Model file for the job. Use its own axes, mm. Face numbers are marked on the shaded views. A direction names the side the tool comes from. Coordinates: 2 decimals unless noted, no trailing zeros. Order: outer loops, then holes, each group sorted by start corner. A loop starts at its lowest first (then second) coordinate and runs counter-clockwise, first axis right, second up. Notation, with made-up numbers: (3.25, 39.5) - (38.25, 39.5) arc R21 cw to (38.25, 43.5) - close; hole circle Ø4 at (24, -4.5). An arc over 180 degrees is marked (long way). Put each result on its own line as item: value. Start each with the question number.
```python
from build123d import *

# Parameters (mm, degrees)
SKETCH1_R           = 11.1125
SKETCH1_R_2         = 4.7625
SKETCH1_R_3         = 14.2875
BOSS_EXTRUDE1_DEPTH = 76.2


with BuildPart() as part:
    # Sketch1 → Boss-Extrude1 (new body)
    with BuildSketch(Plane.XY):
        Polygon((-101.6, 0), (101.6, 0), (130.929393675, 50.8), (130.929393675, 127), (118.229393675, 127), (25.4, 50.8), (-25.4, 50.8), (-118.229393675, 127), (-130.929393675, 127), (-130.929393675, 50.8), align=None)
        with Locations(Location((105.529393675, 76.2, 0), (0, 0, 180))):
            Circle(SKETCH1_R, mode=Mode.SUBTRACT)
        with Locations(Location((92.829393675, 50.8, 0), (0, 0, 180))):
            Circle(SKETCH1_R_2, mode=Mode.SUBTRACT)
        with Locations(Location((92.829393675, 25.4, 0), (0, 0, 180))):
            Circle(SKETCH1_R_2, mode=Mode.SUBTRACT)
        with Locations(Location((0, 25.4, 0), (0, 0, 180))):
            Circle(SKETCH1_R_3, mode=Mode.SUBTRACT)
        with Locations(Location((-92.829393675, 25.4, 0), (0, 0, 180))):
            Circle(SKETCH1_R_2, mode=Mode.SUBTRACT)
        with Locations(Location((-92.829393675, 50.8, 0), (0, 0, 180))):
            Circle(SKETCH1_R_2, mode=Mode.SUBTRACT)
        with Locations(Location((-105.529393675, 76.2, 0), (0, 0, 180))):
            Circle(SKETCH1_R, mode=Mode.SUBTRACT)
    extrude(amount=BOSS_EXTRUDE1_DEPTH)


solid = part.part
```
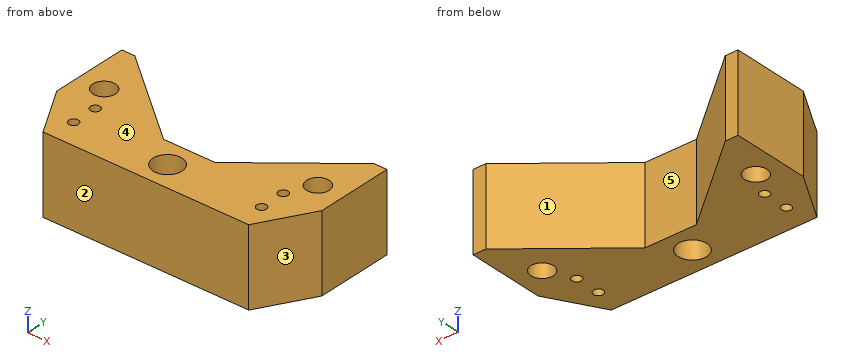
Item 1: Wall check: line 1 along X through (y, z) = (76.2, 38); line 2 along X through (y, z) = (55, 21); line 3 along X through (y, z) = (48, 63.5). Give the ranges that are in metal, low to high.
Item 2: Slice it at B-B, the plane z = 53. Give the cut face in (x, y) (1 decimal).
Item 3: Slice it at A-A, the plane x = 0. Give the cut face in (y, z), plus the area to 3 significant figures.
Item 4: Pull direction X, two halves, no side cores. Call the marked faces 3, 4 and 5: pulls with the +X half, pulls with the -X half, needs draft (parallel to the pull), parting line crosses it, or undercut.
Item 5: Flat gauge pins, fed straight in: pin 1 Ø13.5 at (x, y) = (-105.53, 76.2) entering from +Z; pin 2 Ø2 at (x, z) = (41, 53.5) entering from +Y; pin 3 Ø2 at (y, z) = (24.5, 67.5) entering from +X; pin 4 Ø4 at (x, z) = (46, 19) entering from +Y. Where does each tip first touch, or does it go through?
Item 6: 3-axis set-ups, long thin cutter, end or side, ignore diameter. For the marked faces 1 and 2: which of +Z, -Z, +X, -X, +Y, -Y reach the whole face in a straight line?
Item 7: Slice it at D-D, the plane y = 25.4. Give the cut face in (x, z), plus the area to 3 significant figures.
Item 8: Slice it at C-C, the plane y = 76.2. Give the cut face in (x, z), plus the area to 3 significant figures.
Here are the results:
1. line 1: x = -130.93 to -116.64, -94.42 to -56.34, 56.34 to 94.42, 116.64 to 130.93
1. line 2: x = -130.93 to -95.07, -90.58 to -30.52, 30.52 to 90.58, 95.07 to 130.93
1. line 3: x = -129.31 to -96.68, -88.98 to 88.98, 96.68 to 129.31
2. outline: (-130.9, 50.8) - (-101.6, 0) - (101.6, 0) - (130.9, 50.8) - (130.9, 127) - (118.2, 127) - (25.4, 50.8) - (-25.4, 50.8) - (-118.2, 127) - (-130.9, 127) - close; hole circle Ø22.2 at (-105.5, 76.2); hole circle Ø9.5 at (-92.8, 25.4); hole circle Ø9.5 at (-92.8, 50.8); hole circle Ø28.6 at (0, 25.4); hole circle Ø9.5 at (92.8, 25.4); hole circle Ø9.5 at (92.8, 50.8); hole circle Ø22.2 at (105.5, 76.2)
3. outline: (0, 0) - (11.11, 0) - (11.11, 76.2) - (0, 76.2) - close; (39.69, 0) - (50.8, 0) - (50.8, 76.2) - (39.69, 76.2) - close
3. area: 1,690 mm^2
4. face 3: pulls with the +X half
4. face 4: needs draft
4. face 5: undercut
5. pin 1: passes through
5. pin 2: stops at y = 64.43
5. pin 3: stops at x = 116.32
5. pin 4: stops at y = 69.35
6. face 1: +Z, -Z, +Y
6. face 2: +Z, -Z, +X, -X, -Y
7. outline: (-116.26, 0) - (-97.59, 0) - (-97.59, 76.2) - (-116.26, 76.2) - close; (-88.07, 0) - (-14.29, 0) - (-14.29, 76.2) - (-88.07, 76.2) - close; (14.29, 0) - (88.07, 0) - (88.07, 76.2) - (14.29, 76.2) - close; (97.59, 0) - (116.26, 0) - (116.26, 76.2) - (97.59, 76.2) - close
7. area: 14,100 mm^2
8. outline: (-130.93, 0) - (-116.64, 0) - (-116.64, 76.2) - (-130.93, 76.2) - close; (-94.42, 0) - (-56.34, 0) - (-56.34, 76.2) - (-94.42, 76.2) - close; (56.34, 0) - (94.42, 0) - (94.42, 76.2) - (56.34, 76.2) - close; (116.64, 0) - (130.93, 0) - (130.93, 76.2) - (116.64, 76.2) - close
8. area: 7,980 mm^2
